CAD build for the part. Positions are in the model's coordinates, mm. A direction names the side the tool comes from. Round coordinates to 2 decimals unless told otherwise and drop trailing zeros. Loops run counter-clockwise (first coordinate to the right, second up) from the corner with the lowest first, then second, coordinate; pieces in that order, holes last. Notation, with made-up numbers: M 77,17.5 L 112,17.5 A20 ccw 112,47.5 Z; hole C 66.25,-23.75 d6. An arc over 180 degrees is marked long. Use a Markdown table: item, result. Add a question column.
(1) Band-saw the part on D-D, the plane x = 26. Write the cut outline in (y, z).
(2) Band-saw the part on B-B, the plane x = 12. Write the cut outline in (y, z), and give its area (3 significant figures).
(3) Wall check: L1, parallel to Y at x = 10.5, z = -5.85; L2, parallel to Y at x = -25.5, z = 2.25; L3, parallel to Y at x = 6.5, z = -4. Give the ranges that are in metal, low to high.
(4) Flat gauge pins, fed straight in: P1, Ø1.5, axis at x = 16, y = 4, coming from the -Z side; P2, Ø1.3, axis at x = 0, z = 0, coming from the +Y side. Where does each tip first touch, or does it go through?
(5) Two-plate mould, pull along Y, no slides. Class faces 1 (the face through (0, 9, -3)), 2 (the face through (10, 3, -2.5)), 3 (the face through (13.851, 1, 0)), 4 (the face through (21, 3, -2.5)): released by +Y, released by -Y, zero draft, split by the parting line, or undercut.
(6) Which spindle directions (+Z, -Z, +X, -X, +Y, -Y) get a long thin tool onto all of the face, cutting with end or side? Do faces 5 (the face through (3, 10, 0)), 6 (the face through (0, 5, 7.5)), 7 (the face through (-19.248, 3, 3)), 8 (the face through (-18.5, 3.1, -6)). Say none if no direction does.
(7) Band-saw the part on A-A, the plane z = 3.25. Give the number of separate pieces and of enclosed holes in the cut face, and give its area (3 significant figures).
from build123d import *

# Parameters (mm, degrees)
SKETCH1_W           = 64
SKETCH1_H           = 15
BOSS_EXTRUDE1_DEPTH = 9
CUT_EXTRUDE1_DEPTH  = 10
SKETCH3_R           = 2.5
CUT_EXTRUDE2_DEPTH  = 3
SKETCH4_W           = 6
SKETCH4_H           = 5
BOSS_EXTRUDE2_DEPTH = 2
FILLET1_R           = 1
SKETCH9_W           = 1.20235501
SKETCH9_H           = 15
CUT_EXTRUDE3_DEPTH  = 1.55


with BuildPart() as part:
    # Sketch1 → Boss-Extrude1 (new body)
    with BuildSketch(Plane(origin=(0, 0, 0), x_dir=(1, 0, 0), z_dir=(0, 1, 0))):
        Rectangle(SKETCH1_W, SKETCH1_H)
    extrude(amount=BOSS_EXTRUDE1_DEPTH)

    # Sketch2 → Cut-Extrude1 (cut)
    with BuildSketch(Plane.XY.offset(7.5)):
        Polygon((8.24833395, 4.3), (8.24833395, 1.7), (10.5, 0.4), (12.75166605, 1.7), (12.75166605, 4.3), (10.5, 5.6), align=None)
        Polygon((13.74833395, 4.3), (13.74833395, 1.7), (16, 0.4), (18.25166605, 1.7), (18.25166605, 4.3), (16, 5.6), align=None)
        Polygon((19.24833395, 4.3), (19.24833395, 1.7), (21.5, 0.4), (23.75166605, 1.7), (23.75166605, 4.3), (21.5, 5.6), align=None)
        Polygon((24.74833395, 4.3), (24.74833395, 1.7), (27, 0.4), (29.25166605, 1.7), (29.25166605, 4.3), (27, 5.6), align=None)
        Polygon((2.74833395, 4.3), (2.74833395, 1.7), (5, 0.4), (7.25166605, 1.7), (7.25166605, 4.3), (5, 5.6), align=None)
    cut_extrude1 = extrude(amount=-CUT_EXTRUDE1_DEPTH, mode=Mode.SUBTRACT)

    # Mirror1: Cut-Extrude1 across plane
    add(cut_extrude1.mirror(Plane(origin=(0, 0, 0), x_dir=(0, 0, 1), z_dir=(1, 0, 0))), mode=Mode.SUBTRACT)

    # Sketch3 → Cut-Extrude2 (cut)
    with BuildSketch(Plane(origin=(0, 0, -7.5), x_dir=(-1, 0, 0), z_dir=(0, 0, -1))):
        with Locations((-5, 3)):
            Circle(SKETCH3_R)
        with Locations((-10.5, 3)):
            Circle(SKETCH3_R)
        with Locations((-16, 3)):
            Circle(SKETCH3_R)
        with Locations((-21.5, 3)):
            Circle(SKETCH3_R)
        with Locations((-27, 3)):
            Circle(SKETCH3_R)
    cut_extrude2 = extrude(amount=-CUT_EXTRUDE2_DEPTH, mode=Mode.SUBTRACT)

    # Mirror2: Cut-Extrude2 across plane
    add(cut_extrude2.mirror(Plane(origin=(0, 0, 0), x_dir=(0, 0, 1), z_dir=(1, 0, 0))), mode=Mode.SUBTRACT)

    # Sketch4 → Boss-Extrude2 (add)
    with BuildSketch(Plane(origin=(0, 9, 0), x_dir=(1, 0, 0), z_dir=(0, 1, 0))):
        Rectangle(SKETCH4_W, SKETCH4_H)
    extrude(amount=BOSS_EXTRUDE2_DEPTH)

    # Fillet1
    fillet1_edges = [part.edges().sort_by_distance(p)[0] for p in [
        (-3, 10, 2.5),
        (3, 10, 2.5),
        (3, 10, -2.5),
        (-3, 10, -2.5),
    ]]
    fillet(fillet1_edges, radius=FILLET1_R)

    # Sketch7 → M2 Tapped Hole2 (revolve, cut)
    with BuildSketch(Plane(origin=(0, 11, 0), x_dir=(0, 0, 1), z_dir=(1, 0, 0))):
        Polygon((0, 0), (0, 6), (0.8, 5.519311505), (0.8, 0), align=None)
    revolve(axis=Axis((0, 17.35, 0), (0, -1, 0)), mode=Mode.SUBTRACT)

    # Sketch9 → Cut-Extrude3 (cut)
    with BuildSketch(Plane.XZ):
        with Locations((7.75, 0)):
            Rectangle(SKETCH9_W, SKETCH9_H)
        with Locations((13.25, 0)):
            Rectangle(SKETCH9_W, SKETCH9_H)
        with Locations((18.75, 0)):
            Rectangle(SKETCH9_W, SKETCH9_H)
        with Locations((24.25, 0)):
            Rectangle(SKETCH9_W, SKETCH9_H)
    cut_extrude3 = extrude(amount=-CUT_EXTRUDE3_DEPTH, mode=Mode.SUBTRACT)

    # Mirror3: Cut-Extrude3 across plane
    add(cut_extrude3.mirror(Plane(origin=(0, 0, 0), x_dir=(0, 0, 1), z_dir=(1, 0, 0))), mode=Mode.SUBTRACT)


solid = part.part
Return value:
| question | item | result |
|---|---|---|
| 1 | outline | M 0,-7.5 L 0.71,-7.5 L 0.71,-4.5 L 5.29,-4.5 L 5.29,-7.5 L 9,-7.5 L 9,7.5 L 5.02,7.5 L 5.02,-2.5 L 0.98,-2.5 L 0.98,7.5 L 0,7.5 Z |
| 2 | outline | M 0,-7.5 L 1,-7.5 L 1,-4.5 L 5,-4.5 L 5,-7.5 L 9,-7.5 L 9,7.5 L 4.73,7.5 L 4.73,-2.5 L 1.27,-2.5 L 1.27,7.5 L 0,7.5 Z |
| 2 | area | 88.3 mm^2 |
| 3 | L1 | 0 to 0.5, 5.5 to 9 |
| 3 | L2 | 0 to 1.27, 4.73 to 9 |
| 3 | L3 | 0 to 9 |
| 4 | P1 | z = -4.5 |
| 4 | P2 | y = 5.39 |
| 5 | face 1 | released by +Y |
| 5 | face 2 | undercut |
| 5 | face 3 | zero draft |
| 5 | face 4 | undercut |
| 6 | face 5 | +Z, -Z, +X, +Y |
| 6 | face 6 | +Z, +X, -X, +Y, -Y |
| 6 | face 7 | +Z |
| 6 | face 8 | -Z |
| 7 | separate pieces | 1 |
| 7 | enclosed holes | 10 |
| 7 | area | 385 mm^2 |
